```python
from build123d import *

# Parameters (mm, degrees)
CROQUIS2_W              = 60
CROQUIS2_H              = 50
SALIENTE_EXTRUIR1_DEPTH = 50
CROQUIS3_W              = 60
CROQUIS3_H              = 30
CORTAR_EXTRUIR1_DEPTH   = 35
CROQUIS4_W              = 20
CROQUIS4_H              = 25
CORTAR_EXTRUIR2_DEPTH   = 50
CROQUIS5_W              = 20
CROQUIS5_H              = 30
SALIENTE_EXTRUIR2_DEPTH = 5


with BuildPart() as part:
    # Croquis2 → Saliente-Extruir1 (new body)
    with BuildSketch(Plane.XY):
        Rectangle(CROQUIS2_W, CROQUIS2_H)
    extrude(amount=SALIENTE_EXTRUIR1_DEPTH)

    # Croquis3 → Cortar-Extruir1 (cut)
    with BuildSketch(Plane(origin=(0, 25, 0), x_dir=(1, 0, 0), z_dir=(0, 1, 0))):
        with Locations((0, -35)):
            Rectangle(CROQUIS3_W, CROQUIS3_H)
    extrude(amount=-CORTAR_EXTRUIR1_DEPTH, mode=Mode.SUBTRACT)

    # Croquis4 → Cortar-Extruir2 (cut)
    with BuildSketch(Plane(origin=(0, 0, 0), x_dir=(-1, 0, 0), z_dir=(0, 0, -1))):
        with Locations((0, -12.5)):
            Rectangle(CROQUIS4_W, CROQUIS4_H)
    extrude(amount=-CORTAR_EXTRUIR2_DEPTH, mode=Mode.SUBTRACT)

    # Croquis5 → Saliente-Extruir2 (add)
    with BuildSketch(Plane(origin=(0, -10, 0), x_dir=(1, 0, 0), z_dir=(0, 1, 0))):
        with Locations((20, -35)):
            Rectangle(CROQUIS5_W, CROQUIS5_H)
        with Locations((-20, -35)):
            Rectangle(CROQUIS5_W, CROQUIS5_H)
    extrude(amount=SALIENTE_EXTRUIR2_DEPTH)


solid = part.part
```
Source: CAD feature listing. Evaluate the final solid. Frame: model axes, mm. A direction names the side the tool comes from. Give positions to 0.01 mm unless a question says otherwise; leave off trailing zeros. Write each loop counter-clockwise with the first axis right and the second up, starting at its lowest first coordinate (ties: lowest second). Pieces come first, ordered by that corner, then holes. Notation, with made-up numbers: (85.25, 26) - (115.25, 26) arc R22 cw to (115.25, 64) - close; hole circle Ø11 at (7, 37.25). An arc over 180 degrees is marked (long way). One line per item, written item: value. Start each with the question number.
Q1. Section query C-C, the plane x = -12. Return the cut outline in (y, z).
Q2. Section query D-D, the plane z = 8.5. Return the cut outline in (x, y), then the cut area to 3 significant figures.
Q3. Material intervals for probe 1 along X at (y, z) = (-7, 44); probe 2 along Z at (x, y) = (-7.5, 20.5); probe 3 along Y at (x, z) = (16.5, 46.5), sorted ascending. Write a range as from..to.
Q4. First-contact query: pin 1 Ø10 at (x, z) = (-4, 32) entering from +Y; pin 2 Ø5 at (x, y) = (9, 6.5) entering from +Z; pin 3 Ø6 at (x, z) = (21, 28.5) entering from +Y; pin 4 Ø1 at (x, z) = (2, 20) entering from -Y. Flat tips, straight axial feed; report the tip coordinate or a pass-through.
Q5. Section query B-B, the plane y = -20. Return the cut outline in (x, z), then the cut area to 3 significant figures.
Q6. Section query A-A, the plane z = 36. Return the cut outline in (x, y).
Q7. Set-up query: faces 1 (the face through (10, -13, 25)), 2 (the face through (0, 25, 10)), 3 (the face through (-20, -5, 35)). Return all of +Z, -Z, +X, -X, +Y, -Y with unobstructed straight access to the full face (end or side cutting, diameter ignored); none if empty.
Q8. Draft query along X for faces 4 (the face through (30, -6, 20)), 5 (the face through (0, 10, 20)), 6 (the face through (-10, -13, 25)). Return one class per face: +X half, -X half, draft (parallel to the pull), parting line (faces both ways), or undercut.
Answer:
1. outline: (-25, 0) - (25, 0) - (25, 20) - (-5, 20) - (-5, 50) - (-25, 50) - close
2. outline: (-30, -25) - (-10, -25) - (-10, 0) - (10, 0) - (10, -25) - (30, -25) - (30, 25) - (-30, 25) - close
2. area: 2,500 mm2
3. probe 1: x = -30..-10, 10..30
3. probe 2: z = 0..20
3. probe 3: y = -25..-5
4. pin 1: passes through
4. pin 2: stops at z = 20
4. pin 3: stops at y = -5
4. pin 4: stops at y = 0
5. outline: (-30, 0) - (-10, 0) - (-10, 50) - (-30, 50) - close; (10, 0) - (30, 0) - (30, 50) - (10, 50) - close
5. area: 2,000 mm2
6. outline: (-30, -25) - (-10, -25) - (-10, -5) - (-30, -5) - close; (10, -25) - (30, -25) - (30, -5) - (10, -5) - close
7. face 1: +Z, -Z, -Y
7. face 2: +Z, -Z, +X, -X, +Y
7. face 3: +Z, +X, -X, +Y
8. face 4: +X half
8. face 5: draft
8. face 6: undercut
